Could you check a few things on this model? Use its own coordinates, in mm. Face numbers are marked on the shaded views. A direction names the side the tool comes from. Give positions to 0.01 mm unless a question says otherwise; leave off trailing zeros. Loops run counter-clockwise (first coordinate to the right, second up) from the corner with the lowest first, then second, coordinate; pieces in that order, holes last. Notation, with made-up numbers: (-35.5, 31.5) - (-19.5, 31.5) arc R19 cw to (-19.5, 49.5) - close; hole circle Ø7 at (9, 55). An arc over 180 degrees is marked (long way). Use CSV: the item, a comma, the result in double quotes.
from build123d import *

# Parameters (mm, degrees)
PAD_DEPTH       = 15
POCKET_DEPTH    = 2
SKETCH002_R     = 4
POCKET001_DEPTH = 10
CHAMFER_SIZE    = 1


with BuildPart() as part:
    # Sketch → Pad (new body, symmetric)
    with BuildSketch(Plane.XZ):
        with BuildLine():
            ThreePointArc((1, 25.050126), (0, 45), (-1, 25.050126))
            Line((-1, 0), (-1, 25.050126))
            Line((-1, 0), (-15, 0))
            Line((-15, 0), (-15, 35))
            ThreePointArc((15, 35), (0, 50), (-15, 35))
            Line((15, 35), (15, 0))
            Line((15, 0), (1, 0))
            Line((1, 25.050126), (1, 0))
        make_face()
    extrude(amount=PAD_DEPTH, both=True)

    # Sketch001 (on Face1 of Pad) → Pocket (cut)
    with BuildSketch(Plane(origin=(15, 0, 0), x_dir=(0, 0, 1), z_dir=(1, 0, 0))):
        with BuildLine():
            ThreePointArc((23.228757, -15), (30, 0), (23.228757, 15))
            Line((0, 15), (23.228757, 15))
            Line((0, 15), (0, -15))
            Line((0, -15), (23.228757, -15))
        make_face()
    extrude(amount=-POCKET_DEPTH, mode=Mode.SUBTRACT)

    # Sketch002 (on Face12 of Pocket) → Pocket001 (cut)
    with BuildSketch(Plane(origin=(13, 0, 0), x_dir=(0, 0, 1), z_dir=(1, 0, 0))):
        with Locations((10, 0)):
            Circle(SKETCH002_R)
    extrude(amount=-POCKET001_DEPTH, mode=Mode.SUBTRACT)

    # Chamfer
    chamfer_edges = [part.edges().sort_by_distance(p)[0] for p in [
        (0, -15, 45),
    ]]
    chamfer(chamfer_edges, length=CHAMFER_SIZE)


solid = part.part
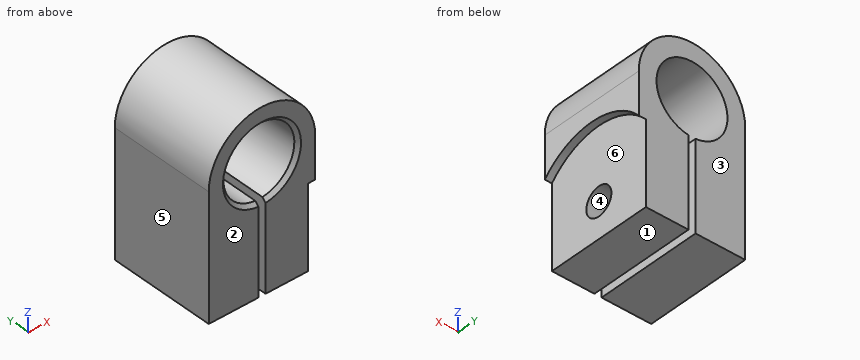
1) I need wall thicknesses on line 1 along X through (y, z) = (6.5, 14); line 2 along Z through (x, y) = (9, 0); line 3 along X through (y, z) = (2, 35). Which ranges of each line are inside material? Lowest first, please.
Answer below:
line 1,"x = -15 to -1, 1 to 13"
line 2,"z = 0 to 6, 14 to 30.64, 39.36 to 47"
line 3,"x = -15 to -10, 10 to 15"
2) Suppose I cut it at D-D (x = 0). Please give me the cut outline in (y, z), plus the area to 4 significant figures.
Answer below:
outline,"(-15, 46) - (-14, 45) - (15, 45) - (15, 50) - (-15, 50) - close"
area,"149.5 mm2"
3) Which directions (+Z, -Z, +X, -X, +Y, -Y) give clear straight access to the entire face, cutting with the end or side of a thin tool? Please do the marked faces 5 and 6.
Answer below:
face 5,"+Z, -Z, -X, +Y, -Y"
face 6,"-Z, +X"
4) Suppose I cut it at A-A (z = 10). Please give me the cut outline in (x, y).
Answer below:
outline,"(-15, -15) - (-1, -15) - (-1, 15) - (-15, 15) - close; (1, -15) - (13, -15) - (13, -4) - (3, -4) - (3, 4) - (13, 4) - (13, 15) - (1, 15) - close"
5) We'd pull the mould along Y, two halves only. Please class the marked faces 1, 2, 3 and 4: +Y half, -Y half, draft (parallel to the pull), parting line (faces both ways), or undercut.
Answer below:
face 1,"draft"
face 2,"-Y half"
face 3,"+Y half"
face 4,"undercut"
6) I'm going to push flat-ended pins straight in: P1, Ø12, axis at x = -7.5, z = 40, coming from the +Y side; P2, Ø9, axis at y = 7.5, z = 22.5, coming from the +X side; P3, Ø8, axis at x = -8.5, y = 8.5, coming from the +Z side; P4, Ø5, axis at y = -9.5, z = 42.5, coming from the +X side. Where does each tip first touch, or does it pass through?
Answer below:
P1,"stops at y = 15"
P2,"stops at x = 13"
P3,"stops at z = 49.31"
P4,"stops at x = 14.14"
7) Suppose I cut it at C-C (z = 15). Please give me the cut outline in (x, y).
Answer below:
outline,"(-15, -15) - (-1, -15) - (-1, 15) - (-15, 15) - close; (1, -15) - (13, -15) - (13, 15) - (1, 15) - close"
8) Suppose I cut it at B-B (y = 0). Please give me the cut outline in (x, z).
Answer below:
outline,"(-15, 0) - (-1, 0) - (-1, 25.05) arc R10 cw (long way) to (1, 25.05) - (1, 0) - (13, 0) - (13, 6) - (3, 6) - (3, 14) - (13, 14) - (13, 30) - (15, 30) - (15, 35) arc R15 ccw to (-15, 35) - close"
